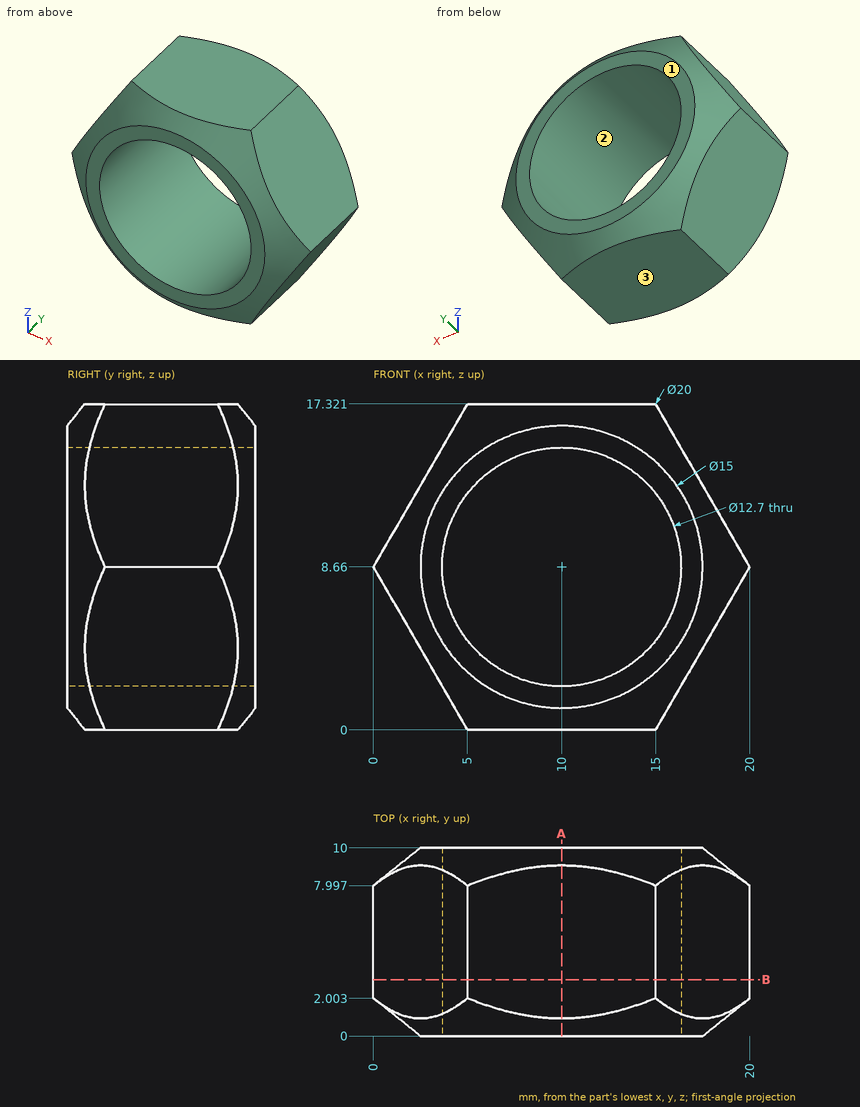
Geometry: see drawing. Coordinates: mm, zero at the bounding-box minimum. Round coordinates to 2 decimals unless told otherwise and drop trailing zeros. Loops run counter-clockwise (first coordinate to the right, second up) from the corner with the lowest first, then second, coordinate; pieces in that order, holes last. Notation, with made-up numbers: (86.25, 22.5) -> (98.25, 22.5) arc R13 cw to (98.25, 41.5) -> close; hole circle Ø10 at (12.25, 70). An arc over 180 degrees is marked (long way). Write each question's results on one line, items separated by ' | '.
1. Ray query, line 1 (Z direction, x = 14.5, y = 3.75); line 2 (X direction, y = 1, z = 12.75) (1 decimal); line 3 (X direction, y = 8.75, z = 5.25) (1 decimal). Return the intervals inside material, ascending. Write a range as from..to.
Geometry results:
line 1: 0..4.18, 13.14..17.32 | line 2: 2.4..5.1, 14.9..17.6 | line 3: 2..4.6, 15.4..18
2. Mould query, pull axis Z, two halves, no side actions, for the marked faces 1, 2 and 3. Classes: +Z half, -Z half, draft (parallel to the pull), parting line (faces both ways), or undercut.
Geometry results:
face 1: draft | face 2: undercut | face 3: -Z half
3. First-contact query: P1, Ø3, axis at y = 2, z = 7, coming from the +X side; P2, Ø1, axis at x = 16.5, y = 6, coming from the -Z side (1 decimal); P3, Ø1, axis at y = 5.5, z = 7, coming from the +X side. Flat tips, straight axial feed; report the tip coordinate or a pass-through.
Geometry results:
P1: x = 19.91 | P2: z = 1.7 | P3: x = 19.33
4. Section A-A (x = 10). Return loops of the section in (y, z).
Geometry results:
outline: (0, 1.16) -> (0.93, 0) -> (9.07, 0) -> (10, 1.16) -> (10, 2.31) -> (0, 2.31) -> close; (0, 15.01) -> (10, 15.01) -> (10, 16.16) -> (9.07, 17.32) -> (0.93, 17.32) -> (0, 16.16) -> close
5. Section B-B (y = 3). Return loops of the section in (x, z).
Geometry results:
outline: (0, 8.66) -> (5, 0) -> (15, 0) -> (20, 8.66) -> (15, 17.32) -> (5, 17.32) -> close; hole circle Ø12.7 at (10, 8.66)
